For this review, take the finished solid that the model builds, in its own axes (mm). Face numbers are marked on the shaded views. A direction names the side the tool comes from. Round coordinates to 2 decimals unless told otherwise and drop trailing zeros. Write each loop counter-clockwise with the first axis right and the second up, starting at its lowest first coordinate (ties: lowest second). Pieces come first, ordered by that corner, then holes. Notation, with made-up numbers: M 83,4 L 140,4 A27 cw 140,25 Z; hole C 8,66 d11. An arc over 180 degrees is marked long. Use one line per item in the form item = value. Start each with the question number.
Item 1: Add section C-C (z = 6.5). State the section outline as (x, y) points, and give its area (3 significant figures).
Item 2: For the marked faces 1 and 2, list the 3-axis set-ups (+Z, -Z, +X, -X, +Y, -Y) from which the entire face can be reached by the end or side of a thin tool; tool diameter is ignored.
Item 3: Add section A-A (y = 0). State the section outline as (x, z) points.
Item 4: For P1, Ø1, axis at y = -4, z = 1, coming from the -X side; P2, Ø1, axis at y = -4, z = 1, coming from the +X side; P3, Ø2, axis at x = 4, z = 4.5, coming from the -Y side, all flat-tipped, find the tip position at first contact; note any pin that passes through.
Item 5: For line 1 (Z direction, x = -2.75, y = 1.25); line 2 (Z direction, x = 4.25, y = 1); line 3 (Y direction, x = -1.75, z = 2.5), list the stretches that pass through material, from the lowest coordinate up. Write a range as [from, to].
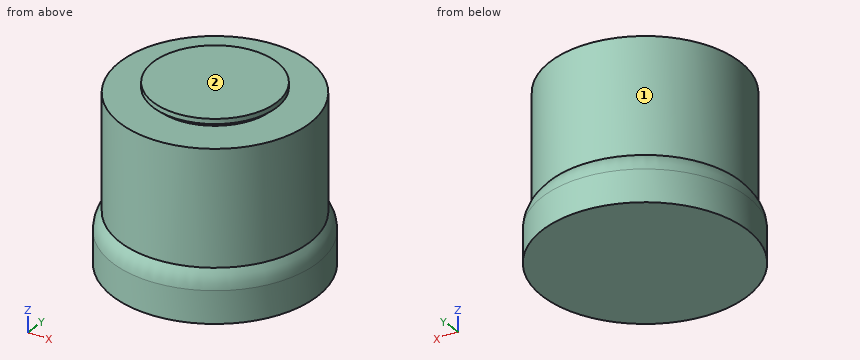
from build123d import *

# Parameters (mm, degrees)
F0_R     = 5.207
F1_DEPTH = 2.54
F2_R     = 4.826
F3_DEPTH = 5.842
F5_R     = 2.8575
F6_DEPTH = 0.254
F7_R     = 3.1496
F8_DEPTH = 0.254


# Not quite as in the source:
# - a fillet or chamfer that OpenCascade refuses, or shapes differently, is made with other operations: its cross-section is extruded or revolved along the edge and cut away or added


with BuildPart() as f1:
    # F0 (on Top) → F1 (new body)
    with BuildSketch(Plane.XY):
        Circle(F0_R)
    extrude(amount=F1_DEPTH)

    # F2 (on face) → F3 (join)
    with BuildSketch(Plane.XY.offset(2.54)):
        Circle(F2_R)
    extrude(amount=F3_DEPTH)

    # F4: fillet of radius 1.27 on 1 edges, made by hand

    # F4_s1 → F4_t2 (revolve, cut)
    with BuildSketch(Plane.XZ):
        with BuildLine():
            ThreePointArc((5.207, 1.6330385896), (5.1078821461, 2.1249074745), (4.826, 2.54))
            Line((4.826, 2.54), (5.207, 2.54))
            Line((5.207, 2.54), (5.207, 1.6330385896))
        make_face()
    revolve(axis=Axis((0, 0, 2.54), (0, 0, 1)), mode=Mode.SUBTRACT)

    # F5 (on face) → F6 (join)
    with BuildSketch(Plane.XY.offset(8.382)):
        Circle(F5_R)
    extrude(amount=F6_DEPTH)

    # F7 (on face) → F8 (join)
    with BuildSketch(Plane.XY.offset(8.636)):
        Circle(F7_R)
    extrude(amount=F8_DEPTH)


solid = f1.part
Calculated:
q1.outline = C 0,0 d9.65
q1.area = 73.2 mm^2
q2.face_1 = +Z
q2.face_2 = +Z, +X, -X, +Y, -Y
q3.outline = M -5.21,0 L 5.21,0 L 5.21,1.63 A1.27 ccw 4.83,2.54 L 4.83,8.38 L 2.86,8.38 L 2.86,8.64 L 3.15,8.64 L 3.15,8.89 L -3.15,8.89 L -3.15,8.64 L -2.86,8.64 L -2.86,8.38 L -4.83,8.38 L -4.83,2.54 A1.27 ccw -5.21,1.63 Z
q4.P1 = -3.86
q4.P2 = 3.86
q4.P3 = -3.78
q5.line_1 = [0, 8.38], [8.64, 8.89]
q5.line_2 = [0, 8.38]
q5.line_3 = [-4.54, 4.54]
